```python
from build123d import *

# Parameters (mm, degrees)
F3_DEPTH   = 6
F5_D       = 3.3
F5_ON_F1_D = 3.3
F6_DEPTH   = 2
F7_D       = 11


with BuildPart() as f3:
    # F2 (on Top) → F3 (new body)
    with BuildSketch(Plane.XY):
        with BuildLine():
            Line((57.1005050634, 76.8994949366), (9.2390693497, 29.0380592229))
            Line((9.2390693497, 29.0380592229), (-10.8754739071, 29.0380592229))
            Line((-10.8754739071, 29.0380592229), (-57.1005050634, 76.8994949366))
            ThreePointArc((-57.1005050634, 76.8994949366), (-87.7279220614, 87.7279220614), (-76.8994949366, 57.1005050634))
            Line((-76.8994949366, 57.1005050634), (-29.7989898732, 10))
            Line((-29.7989898732, 10), (-29.7989898732, -10))
            Line((-29.7989898732, -10), (-76.8994949366, -57.1005050634))
            ThreePointArc((-76.8994949366, -57.1005050634), (-87.7279220614, -87.7279220614), (-57.1005050634, -76.8994949366))
            Line((-57.1005050634, -76.8994949366), (-20.217323358, -40.0163132312))
            Line((-20.217323358, -40.0163132312), (20.217323358, -40.0163132312))
            Line((20.217323358, -40.0163132312), (57.1005050634, -76.8994949366))
            ThreePointArc((57.1005050634, -76.8994949366), (87.7279220614, -87.7279220614), (76.8994949366, -57.1005050634))
            Line((76.8994949366, -57.1005050634), (29.7989898732, -10))
            Line((29.7989898732, -10), (29.7989898732, 10))
            Line((29.7989898732, 10), (76.8994949366, 57.1005050634))
            ThreePointArc((76.8994949366, 57.1005050634), (87.7279220614, 87.7279220614), (57.1005050634, 76.8994949366))
        make_face()
        with BuildLine():
            Line((-14.25, 10), (-14.25, -10))
            ThreePointArc((-14.25, -10), (-15.25, -11), (-16.25, -10))
            Line((-16.25, -10), (-16.25, 10))
            ThreePointArc((-16.25, 10), (-15.25, 11), (-14.25, 10))
        make_face(mode=Mode.SUBTRACT)
        with BuildLine():
            Line((16.25, 10), (16.25, -10))
            ThreePointArc((16.25, -10), (15.25, -11), (14.25, -10))
            Line((14.25, -10), (14.25, 10))
            ThreePointArc((14.25, 10), (15.25, 11), (16.25, 10))
        make_face(mode=Mode.SUBTRACT)
    extrude(amount=F3_DEPTH)

    # F5 (through all)
    with Locations(Plane(origin=(0, 0, 0), x_dir=(1, 0, 0), z_dir=(0, 0, -1))):
        with Locations((-83, -75), (-75, -84.5), (-67, -75), (-75, -65.5), (-75, 65.5), (-83, 75), (-75, 84.5), (-67, 75), (67, 75), (75, 65.5), (83, 75), (75, 84.5), (75, -65.5), (67, -75), (75, -84.5), (83, -75)):
            Hole(F5_D / 2)

    # F5 on F1 (through all)
    with Locations(Plane(origin=(0, 0, 0), x_dir=(1, 0, 0), z_dir=(0, 0, -1))):
        with Locations((-15.25, -15.25), (15.25, -15.25), (15.25, 15.25), (-15.25, 15.25), (0, 33.0380592229)):
            Hole(F5_ON_F1_D / 2)

    # F4 (on face) → F6 (cut)
    with BuildSketch(Plane.XY.offset(6)):
        with BuildLine():
            Line((-11.7243497964, 27.0380592229), (-59.0326143525, 76.0210757))
            ThreePointArc((-59.0326143525, 76.0210757), (-86.3204761024, 86.3069368449), (-76.0019666007, 59.0314038522))
            Line((-76.0019666007, 59.0314038522), (-27.7989898732, 10.8284271247))
            Line((-27.7989898732, 10.8284271247), (-27.7989898732, -10.8284271247))
            Line((-27.7989898732, -10.8284271247), (-76.0019666007, -59.0314038522))
            ThreePointArc((-76.0019666007, -59.0314038522), (-86.313708499, -86.313708499), (-59.0314038522, -76.0019666007))
            Line((-59.0314038522, -76.0019666007), (-21.0457504827, -38.0163132312))
            Line((-21.0457504827, -38.0163132312), (21.0457504827, -38.0163132312))
            Line((21.0457504827, -38.0163132312), (59.0314038522, -76.0019666007))
            ThreePointArc((59.0314038522, -76.0019666007), (86.313708499, -86.313708499), (76.0019666007, -59.0314038522))
            Line((76.0019666007, -59.0314038522), (27.7989898732, -10.8284271247))
            Line((27.7989898732, -10.8284271247), (27.7989898732, 10.8284271247))
            Line((27.7989898732, 10.8284271247), (76.0019666007, 59.0314038522))
            ThreePointArc((76.0019666007, 59.0314038522), (86.313708499, 86.313708499), (59.0314038522, 76.0019666007))
            Line((59.0314038522, 76.0019666007), (10.0674964744, 27.0380592229))
            Line((10.0674964744, 27.0380592229), (-11.7243497964, 27.0380592229))
        make_face()
    extrude(amount=-F6_DEPTH, mode=Mode.SUBTRACT)

    # F7 (through all)
    with Locations(Plane(origin=(0, 0, 0), x_dir=(1, 0, 0), z_dir=(0, 0, -1))):
        with Locations((-75, -75), (75, -75), (-75, 75), (75, 75)):
            Hole(F7_D / 2)


solid = f3.part
```
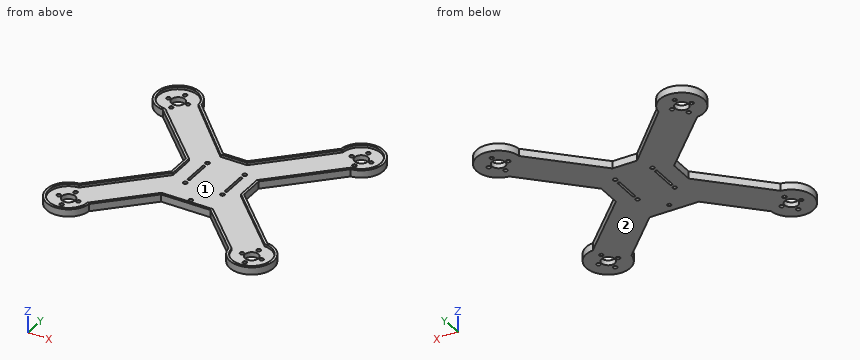
Geometry check sheet. Reference: the model listing, model coordinates, mm. Face numbers are marked on the shaded views. Coordinates: 2 decimals unless noted, no trailing zeros. Write each loop counter-clockwise with the first axis right and the second up, starting at its lowest first coordinate (ties: lowest second). Pieces come first, ordered by that corner, then holes. Notation, with made-up numbers: M 18,-13.75 L 25,-13.75 A12 cw 25,-9.75 Z; hole C -9.75,-11.75 d1. An arc over 180 degrees is marked long. One line per item, written item: value. Start each with the question number.
(1) Sectioned sample at A-A, the plane x = -63. Enter the section's corners in (y, z), and give its area (3 significant figures).
(2) Sectioned sample at C-C, the plane z = 2.2. State how many separate pieces and enclosed holes the cut face has, and give its area (3 significant figures).
(3) Sectioned sample at B-B, the plane y = 45.5. Enter the section's corners in (x, z).
(4) Depth check by flat-ended pin: pin 1 (5.5 mm diameter, centred on x = -15.25, y = 15.25, fed in from +Z); pin 2 (3 mm diameter, centred on x = 58.5, z = 2.5, fed in from +Y); pin 3 (1.8 mm diameter, centred on x = 2.5, z = 3, fed in from +Y). Enter the tip coordinate at first touch or a pass-through.
(5) Release check for a two-part mould opening along Y. For the marked faces 1 and 2 record: released by +Y, released by -Y, zero draft, split by the parting line, or undercut.
(6) Scan lines: line 1 along X through (y, z) = (7, 4.1); line 2 along X through (y, z) = (32.5, 5.55); line 3 along Y through (x, z) = (57, 4.15). Record each from-to range of solid material in increasing order. Write a range as [from, to].
Filled sheet:
1. outline: M -88.42,0 L -43.2,0 L -43.2,6 L -46.03,6 L -46.03,4 L -85.58,4 L -85.58,6 L -88.42,6 Z; M 43.2,0 L 88.42,0 L 88.42,6 L 85.58,6 L 85.58,4 L 46.03,4 L 46.03,6 L 43.2,6 Z
1. area: 384 mm²
2. separate pieces: 1
2. enclosed holes: 27
2. area: 13,400 mm²
3. outline: M -65.3,0 L -26.77,0 L -26.77,6 L -29.56,6 L -29.56,4 L -62.47,4 L -62.47,6 L -65.3,6 Z; M 25.7,0 L 65.3,0 L 65.3,6 L 62.47,6 L 62.47,4 L 28.53,4 L 28.53,6 L 25.7,6 Z
4. pin 1: z = 4
4. pin 2: y = 84.95
4. pin 3: y = 29.04
5. face 1: undercut
5. face 2: zero draft
6. line 1: [-29.8, -27.8], [27.8, 29.8]
6. line 2: [-52.3, -49.47], [-17, -14.22], [12.7, 15.53], [49.47, 52.3]
6. line 3: [-76.8, -73.97], [-40.03, -37.2], [37.2, 40.03], [73.97, 76.8]
